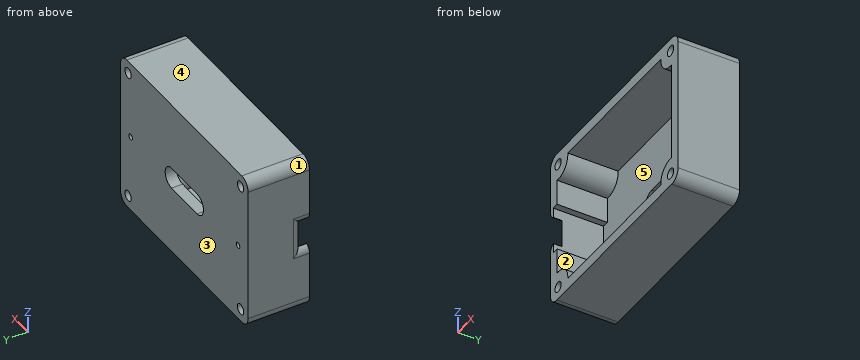
```python
from build123d import *

# Parameters (mm, degrees)
SKETCH1_W           = 80
SKETCH1_H           = 59
BOSS_EXTRUDE1_DEPTH = 23
SKETCH2_R           = 1.95
CUT_EXTRUDE1_DEPTH  = 23
SHELL2_T            = -4.15
CUT_EXTRUDE2_DEPTH  = 23
SKETCH4_W           = 10
SKETCH4_H           = 3
CUT_EXTRUDE3_DEPTH  = 23
FILLET1_R           = 4
FILLET2_R           = 3
SKETCH5_R           = 1.08
CUT_EXTRUDE4_DEPTH  = 10
SKETCH6_W           = 2.4
SKETCH6_H           = 18
CUT_EXTRUDE5_DEPTH  = 18.85


with BuildPart() as part:
    # Sketch1 → Boss-Extrude1 (new body)
    with BuildSketch(Plane(origin=(0, 0, 0), x_dir=(1, 0, 0), z_dir=(0, 1, 0))):
        Rectangle(SKETCH1_W, SKETCH1_H)
    extrude(amount=BOSS_EXTRUDE1_DEPTH)

    # Sketch2 → Cut-Extrude1 (cut)
    with BuildSketch(Plane(origin=(0, 23, 0), x_dir=(1, 0, 0), z_dir=(0, 1, 0))):
        with Locations(Location((35.25, 24.75, 0), (0, 0, 270))):
            Circle(SKETCH2_R)
        with Locations(Location((35.25, -24.75, 0), (0, 0, 270))):
            Circle(SKETCH2_R)
        with Locations(Location((-35.25, 24.75, 0), (0, 0, 270))):
            Circle(SKETCH2_R)
        with Locations(Location((-35.25, -24.75, 0), (0, 0, 270))):
            Circle(SKETCH2_R)
    extrude(amount=-CUT_EXTRUDE1_DEPTH, mode=Mode.SUBTRACT)

    # Shell2
    shell2_openings = [part.faces().sort_by_distance(p)[0] for p in [
        (0, 0, 0),
    ]]
    offset(amount=SHELL2_T, openings=shell2_openings)

    # Sketch3 → Cut-Extrude2 (cut)
    with BuildSketch(Plane(origin=(0, 23, 0), x_dir=(1, 0, 0), z_dir=(0, 1, 0))):
        with BuildLine():
            Line((8, -4), (-8, -4))
            ThreePointArc((-8, -4), (-12, 0), (-8, 4))
            Line((-8, 4), (8, 4))
            ThreePointArc((8, 4), (12, 0), (8, -4))
        make_face()
    extrude(amount=-CUT_EXTRUDE2_DEPTH, mode=Mode.SUBTRACT)

    # Sketch4 → Cut-Extrude3 (cut)
    with BuildSketch(Plane.ZY.offset(40)):
        with Locations((0, 1.5)):
            Rectangle(SKETCH4_W, SKETCH4_H)
    extrude(amount=-CUT_EXTRUDE3_DEPTH, mode=Mode.SUBTRACT)

    # Fillet1
    fillet1_edges = [part.edges().sort_by_distance(p)[0] for p in [
        (40, 11.5, 29.5),
        (-40, 11.5, 29.5),
        (-40, 11.5, -29.5),
        (40, 11.5, -29.5),
    ]]
    fillet(fillet1_edges, radius=FILLET1_R)

    # Fillet2
    fillet2_edges = [part.edges().sort_by_distance(p)[0] for p in [
        (-40, 1.5, -5),
        (-40, 1.5, 5),
        (-40, 3, 0),
    ]]
    fillet(fillet2_edges, radius=FILLET2_R)

    # Sketch5 → Cut-Extrude4 (cut)
    with BuildSketch(Plane(origin=(0, 23, 0), x_dir=(1, 0, 0), z_dir=(0, 1, 0))):
        with Locations(Location((33.67, 0, 0), (0, 0, 270))):
            Circle(SKETCH5_R)
        with Locations(Location((-33.67, 0, 0), (0, 0, 270))):
            Circle(SKETCH5_R)
    extrude(amount=-CUT_EXTRUDE4_DEPTH, mode=Mode.SUBTRACT)

    # Sketch6 → Cut-Extrude5 (cut)
    with BuildSketch(Plane(origin=(0, 0, 0), x_dir=(-1, 0, 0), z_dir=(0, -1, 0))):
        with Locations((37.05, 0)):
            Rectangle(SKETCH6_W, SKETCH6_H)
    extrude(amount=-CUT_EXTRUDE5_DEPTH, mode=Mode.SUBTRACT)


solid = part.part
```
Work out the finished part from the listing and answer in its coordinate system (mm). Face numbers are marked on the shaded views. A direction names the side the tool comes from. Give positions to 0.01 mm unless a question says otherwise; leave off trailing zeros. Write each loop counter-clockwise with the first axis right and the second up, starting at its lowest first coordinate (ties: lowest second). Pieces come first, ordered by that corner, then holes.
(1) The part is cut by section A-A on x = 6.5. Write down the section's boundary in (y, z), plus the area to 3 significant figures.
Final values:
outline: (0, -29.5) - (23, -29.5) - (23, -4) - (18.85, -4) - (18.85, -25.35) - (0, -25.35) - close; (0, 25.35) - (18.85, 25.35) - (18.85, 4) - (23, 4) - (23, 29.5) - (0, 29.5) - close
area: 368 mm2
(2) The mould has two halves that part along Z. Classify the marked faces 3, 4 and 5: pulls with the +Z half, pulls with the -Z half, needs draft (parallel to the pull), parting line crosses it, or undercut.
Final values:
face 3: needs draft
face 4: pulls with the +Z half
face 5: undercut
(3) The part is cut by section B-B on y = 7.25. Write down the section's boundary in (x, z).
Final values:
outline: (-40, -25.5) arc R4 ccw to (-36, -29.5) - (36, -29.5) arc R4 ccw to (40, -25.5) - (40, 25.5) arc R4 ccw to (36, 29.5) - (-36, 29.5) arc R4 ccw to (-40, 25.5) - close; hole (-38.25, -9) - (-35.85, -9) - (-35.85, -18.68) arc R6.1 cw to (-29.18, -25.35) - (29.18, -25.35) arc R6.1 cw to (35.85, -18.68) - (35.85, 18.68) arc R6.1 cw to (29.18, 25.35) - (-29.18, 25.35) arc R6.1 cw to (-35.85, 18.68) - (-35.85, 9) - (-38.25, 9) - close; hole circle Ø3.9 at (-35.25, -24.75); hole circle Ø3.9 at (-35.25, 24.75); hole circle Ø3.9 at (35.25, -24.75); hole circle Ø3.9 at (35.25, 24.75)
(4) Straight lines are drawn through the part: line 1 (X direction, y = 10.75, z = 24.75); line 2 (X direction, y = 20.55, z = 0); line 3 (Z direction, x = 26, y = 16.5). For each, find the intervals that lie inside material, in ascending order.
Final values:
line 1: x = -40 to -37.2, -33.3 to -29.15, 29.15 to 33.3, 37.2 to 40
line 2: x = -40 to -34.75, -32.59 to -12, 12 to 32.59, 34.75 to 40
line 3: z = -29.5 to -25.35, 25.35 to 29.5
(5) The part is cut by section C-C on z = 0. Write down the section's boundary in (x, y), plus the area to 3 significant figures.
Final values:
outline: (-40, 6) arc R3 ccw to (-38.25, 3.27) - (-38.25, 18.85) - (-34.75, 18.85) - (-34.75, 23) - (-40, 23) - close; (-32.59, 18.85) - (-12, 18.85) - (-12, 23) - (-32.59, 23) - close; (12, 18.85) - (32.59, 18.85) - (32.59, 23) - (12, 23) - close; (34.75, 18.85) - (35.85, 18.85) - (35.85, 0) - (40, 0) - (40, 23) - (34.75, 23) - close
area: 319 mm2
(6) Flat-ended cylindrical pins translate along their axes: pin 1 Ø1.5 at (x, z) = (1, -3) entering from +Y; pin 2 Ø2.5 at (x, y) = (-37.5, 8) entering from -Z; pin 3 Ø15 at (x, z) = (17, -3.5) entering from -Y. Find the tip coordinate at first contact, or state that the pin passes through.
Final values:
pin 1: passes through
pin 2: stops at z = -29.49
pin 3: stops at y = 18.85
(7) The part is cut by section D-D on y = 2. Write down the section's boundary in (x, z), plus the area to 3 significant figures.
Final values:
outline: (-40, -25.5) arc R4 ccw to (-36, -29.5) - (36, -29.5) arc R4 ccw to (40, -25.5) - (40, 25.5) arc R4 ccw to (36, 29.5) - (-36, 29.5) arc R4 ccw to (-40, 25.5) - (-40, 8) arc R3 ccw to (-38.25, 5.27) - (-38.25, 9) - (-35.85, 9) - (-35.85, 18.68) arc R6.1 ccw to (-29.18, 25.35) - (29.18, 25.35) arc R6.1 ccw to (35.85, 18.68) - (35.85, -18.68) arc R6.1 ccw to (29.18, -25.35) - (-29.18, -25.35) arc R6.1 ccw to (-35.85, -18.68) - (-35.85, -9) - (-38.25, -9) - (-38.25, -5.27) arc R3 ccw to (-40, -8) - close; hole circle Ø3.9 at (-35.25, -24.75); hole circle Ø3.9 at (-35.25, 24.75); hole circle Ø3.9 at (35.25, -24.75); hole circle Ø3.9 at (35.25, 24.75)
area: 1,110 mm2
(8) Which of the six approach directions +Z, -Z, +X, -X, +Y, -Y give full straight-line access (tool end or side, diameter ignored) to the marked faces 1 and 2?
Final values:
face 1: +Z, -X, +Y, -Y
face 2: -Y
